The drawing under review shows one solid part. Ordinate dimensions are in mm from its lowest x, y, z. A direction names the side the tool comes from. Give positions to 0.01 mm unless a question says otherwise; leave off trailing zeros. Write each loop counter-clockwise with the first axis right and the second up, starting at its lowest first coordinate (ties: lowest second). Pieces come first, ordered by that corner, then holes. Notation, with made-up numbers: (27, -2.5) -> (85, -2.5) arc R22 ccw to (85, 11.5) -> close; hole circle Ø2 at (18, 64). An arc over 180 degrees is marked (long way). Use CSV: the item, a comma, the result in double quotes.
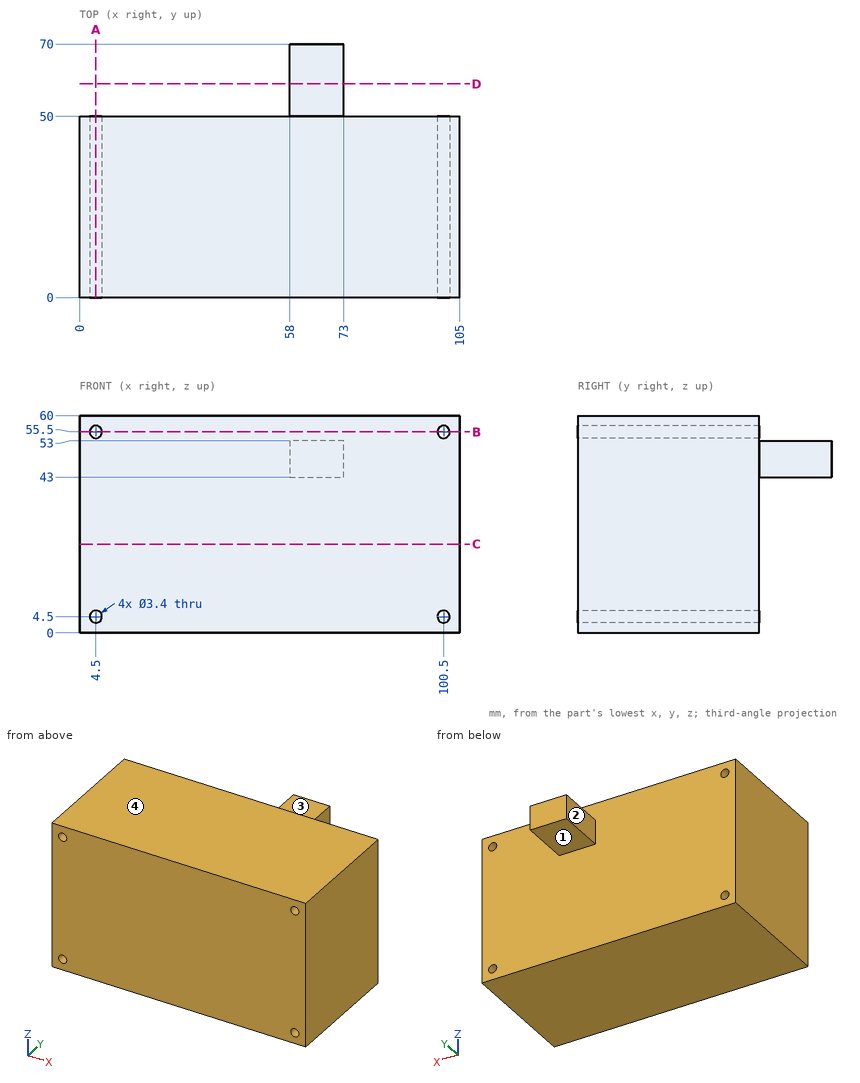
(1) Tool access review of the marked faces 1, 2, 3 and 4: name each direction out of +Z, -Z, +X, -X, +Y, -Y from which nothing blocks a thin tool from reaching the whole face with its end or side.
Established:
face 1,"-Z, +X, -X, +Y"
face 2,"+Z, -Z, -X, +Y"
face 3,"+Z, +X, -X, +Y"
face 4,"+Z, +X, -X, +Y, -Y"
(2) Take a section at C-C (z = 24.5). Write out the cut boundary in (x, y).
Established:
outline,"(0, 0) -> (105, 0) -> (105, 50) -> (0, 50) -> close"
(3) Take a section at D-D (y = 59). Write out the cut boundary in (x, z).
Established:
outline,"(58, 43) -> (73, 43) -> (73, 53) -> (58, 53) -> close"
(4) Take a section at B-B (z = 55.5). Write out the cut boundary in (x, y), then the cut area to 3 significant figures.
Established:
outline,"(0, 0) -> (2.8, 0) -> (2.8, 50) -> (0, 50) -> close; (6.2, 0) -> (98.8, 0) -> (98.8, 50) -> (6.2, 50) -> close; (102.2, 0) -> (105, 0) -> (105, 50) -> (102.2, 50) -> close"
area,"4,910 mm2"
(5) For line 1 along X through (y, z) = (13.5, 4.5); line 2 along Z through (x, y) = (4.5, 16); line 3 along X through (y, z) = (26, 4), list the stretches that pass through material, from the lowest coordinate up. Write a range as [from, to].
Established:
line 1,"x = [0, 2.8], [6.2, 98.8], [102.2, 105]"
line 2,"z = [0, 2.8], [6.2, 53.8], [57.2, 60]"
line 3,"x = [0, 2.88], [6.12, 98.88], [102.12, 105]"
(6) Take a section at A-A (x = 4.5). Write out the cut boundary in (y, z), then the cut area to 3 significant figures.
Established:
outline,"(0, 0) -> (50, 0) -> (50, 2.8) -> (0, 2.8) -> close; (0, 6.2) -> (50, 6.2) -> (50, 53.8) -> (0, 53.8) -> close; (0, 57.2) -> (50, 57.2) -> (50, 60) -> (0, 60) -> close"
area,"2,660 mm2"
(7) Clearance check with flat-ended pins moving along their axes: pin 1 (8 mm diameter, centred on y = 63, z = 46.5, fed in from +X); pin 2 (4 mm diameter, centred on x = 52.5, z = 33.5, fed in from +Y); pin 3 (16.5 mm diameter, centred on x = 67, y = 60, fed in from +Z). State where each tip first meets the part, or that it passes through.
Established:
pin 1,"stops at x = 73"
pin 2,"stops at y = 50"
pin 3,"stops at z = 53"
